from build123d import *

# Parameters (mm, degrees)
SKETCH_6_W          = 80
SKETCH_6_H          = 31
EXTRUDE_1_DEPTH     = 85
SKETCH_8_W          = 18
SKETCH_8_H          = 30
CUT_EXTRUDE_1_DEPTH = 100
SKETCH_9_W          = 44
SKETCH_9_H          = 30
EXTRUDE_3_DEPTH     = 5
CUT_EXTRUDE_2_DEPTH = 110


with BuildPart() as part:
    # 草图6 → 凸台-拉伸1 (new body)
    with BuildSketch(Plane.XY):
        with Locations((40, -15.5)):
            Rectangle(SKETCH_6_W, SKETCH_6_H)
    extrude(amount=EXTRUDE_1_DEPTH)

    # 草图8 → 切除-拉伸1 (cut)
    with BuildSketch(Plane(origin=(0, 0, 0), x_dir=(1, 0, 0), z_dir=(0, 1, 0))):
        with Locations((71, -70)):
            Rectangle(SKETCH_8_W, SKETCH_8_H)
        with Locations((9, -70)):
            Rectangle(SKETCH_8_W, SKETCH_8_H)
    extrude(amount=-CUT_EXTRUDE_1_DEPTH, mode=Mode.SUBTRACT)

    # 草图9 → 凸台-拉伸3 (add)
    with BuildSketch(Plane(origin=(0, 0, 0), x_dir=(1, 0, 0), z_dir=(0, 1, 0))):
        Polygon((18, -55), (62, -55), (80, -55), (80, 0), (0, 0), (0, -55), align=None)
        with Locations((40, -70)):
            Rectangle(SKETCH_9_W, SKETCH_9_H)
    extrude(amount=EXTRUDE_3_DEPTH)

    # 草图10 → 切除-拉伸2 (cut)
    with BuildSketch(Plane.XZ.offset(31)):
        Polygon((10, 0), (55, 0), (55, 2), (58.5, 5.5), (10, 5.5), align=None)
        with BuildLine():
            Line((39.91937897, 81.354169844), (42.016320752, 79.468982831))
            Line((42.016320752, 79.468982831), (54.182900006, 79.468982831))
            ThreePointArc((54.182900006, 79.468982831), (55.737637047, 76.92860624), (56.279841788, 74))
            Line((56.279841788, 74), (62, 74))
            Line((62, 74), (62, 85))
            Line((62, 85), (18, 85))
            Line((18, 85), (18, 74))
            Line((18, 74), (39.91937897, 74))
            ThreePointArc((39.91937897, 74), (39.969784262, 74.906704585), (40.120378957, 75.802235229))
            Line((40.120378957, 75.802235229), (37.090951845, 78.52574272))
            Line((37.090951845, 78.52574272), (39.91937897, 81.354169844))
        make_face()
    extrude(amount=-CUT_EXTRUDE_2_DEPTH, mode=Mode.SUBTRACT)


solid = part.part
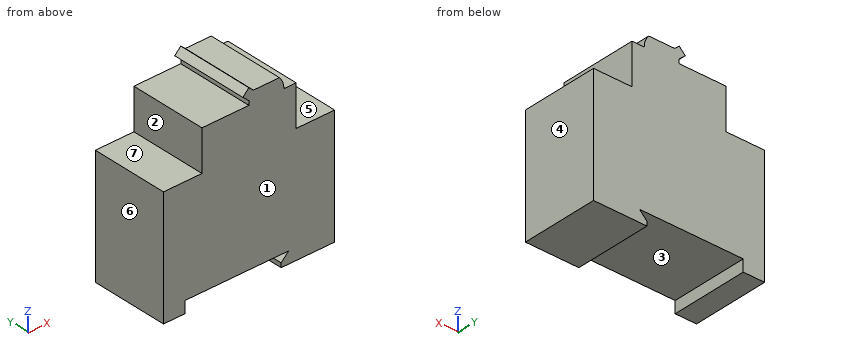
Geometry: final body of the model. Coordinates: model frame, mm. Face numbers are marked on the shaded views. A direction names the side the tool comes from. Give positions to 0.01 mm unless a question says otherwise; leave off trailing zeros. Write each loop counter-clockwise with the first axis right and the second up, starting at its lowest first coordinate (ties: lowest second). Pieces come first, ordered by that corner, then holes. Notation, with made-up numbers: (44.5, 63) -> (69.5, 63) arc R20 ccw to (69.5, 88) -> close; hole circle Ø8 at (-2, 72.25). An arc over 180 degrees is marked (long way). Answer as a JSON object with one key per item and string values.
1. Cut plane B-B on x = 66.5. Output: boundary loops of the cut face in (y, z), and give its area (3 significant figures).
Ans:
{"outline": "(-31, 0) -> (5, 0) -> (5, 55) -> (-31, 55) -> close", "area": "1,980 mm^2"}
2. Cut plane C-C on x = 52. Output: boundary loops of the cut face in (y, z), and give its area (3 significant figures).
Ans:
{"outline": "(-31, 5.5) -> (5, 5.5) -> (5, 79.47) -> (-31, 79.47) -> close", "area": "2,660 mm^2"}
3. Ray query, probe 1 along Z at (x, y) = (48, -6); probe 2 along Z at (x, y) = (56.5, -6); probe 3 along Z at (x, y) = (22.5, -14.5). Return the intervals inside material, ascending. Write a range as from..to.
Ans:
{"probe 1": "z = 5.5..79.47", "probe 2": "z = 0..3.5, 5.5..74", "probe 3": "z = 5.5..74"}
4. Cut plane A-A on y = -13.5. Output: boundary loops of the cut face in (x, z).
Ans:
{"outline": "(0, 0) -> (10, 0) -> (10, 5.5) -> (58.5, 5.5) -> (55, 2) -> (55, 0) -> (80, 0) -> (80, 55) -> (62, 55) -> (62, 74) -> (56.28, 74) arc R8.18 ccw to (54.18, 79.47) -> (42.02, 79.47) -> (39.92, 81.35) -> (37.09, 78.53) -> (40.12, 75.8) arc R8.18 ccw to (39.92, 74) -> (18, 74) -> (18, 55) -> (0, 55) -> close"}
5. Mould query, pull axis X, two halves, no side actions, for the marked faces 1, 2, 3 and 4. Classes: pulls with the +X half, pulls with the -X half, needs draft (parallel to the pull), parting line crosses it, or undercut.
Ans:
{"face 1": "needs draft", "face 2": "pulls with the -X half", "face 3": "undercut", "face 4": "pulls with the +X half"}
6. Contact query for flat-ended pins moving along their axis: pin 1 (6.5 mm diameter, centred on x = 34, y = -20.5, fed in from +Z); pin 2 (1.5 mm diameter, centred on x = 35.5, y = -15.5, fed in from -Z); pin 3 (6 mm diameter, centred on x = 51, y = -8, fed in from +Z). Output: stop coordinate, or through.
Ans:
{"pin 1": "stops at z = 78.68", "pin 2": "stops at z = 5.5", "pin 3": "stops at z = 79.47"}
7. Access query for the marked faces 5, 6 and 7. Directions: +Z, -Z, +X, -X, +Y, -Y. A direction counts if a zero-diameter tool reaches every point of the face in a straight line with its end or side. Return the directions, or none.
Ans:
{"face 5": "+Z, +X, +Y, -Y", "face 6": "+Z, -Z, -X, +Y, -Y", "face 7": "+Z, -X, +Y, -Y"}
